```python
from build123d import *

# Parameters (mm, degrees)
F1_DEPTH = 12
F2_DEPTH = 8
F3_DEPTH = 5
F4_D     = 1.25


with BuildPart() as f1:
    # F0 (on Front) → F1 (new body)
    with BuildSketch(Plane.XZ):
        with BuildLine():
            Line((10.99224894, 5.3214330306), (12.920611769, 7.61956636))
            ThreePointArc((12.920611769, 7.61956636), (10.5696440554, 10.6434310512), (7.529497646, 12.9733058701))
            Line((7.529497646, 12.9733058701), (5.1924112184, 10.1880747237))
            Line((5.1924112184, 10.1880747237), (10.99224894, 5.3214330306))
        make_face()
        Polygon((3.2635182233, -3.8893095672), (10.99224894, 5.3214330306), (5.1924112184, 10.1880747237), (0, 4), (0, 0), align=None)
        Polygon((-3.939231012, -0.6945927107), (0, 0), (0, 4), align=None)
        Polygon((-3.3318045088, -11.7493091275), (3.2635182233, -3.8893095672), (0, 0), (-3.939231012, -0.6945927107), (-9.1316422304, -6.8826674344), align=None)
        with BuildLine():
            ThreePointArc((-11.4687286581, -9.6678985807), (-8.6463339891, -12.2572798185), (-5.2601673378, -14.0474424568))
            Line((-5.2601673378, -14.0474424568), (-3.3318045088, -11.7493091275))
            Line((-3.3318045088, -11.7493091275), (-9.1316422304, -6.8826674344))
            Line((-9.1316422304, -6.8826674344), (-11.4687286581, -9.6678985807))
        make_face()
    extrude(amount=F1_DEPTH)

    # F0 (on Front) → F2 (cut)
    with BuildSketch(Plane.XZ):
        Polygon((-3.939231012, -0.6945927107), (0, 0), (0, 4), align=None)
        Polygon((3.2635182233, -3.8893095672), (10.99224894, 5.3214330306), (5.1924112184, 10.1880747237), (0, 4), (0, 0), align=None)
        Polygon((-3.3318045088, -11.7493091275), (3.2635182233, -3.8893095672), (0, 0), (-3.939231012, -0.6945927107), (-9.1316422304, -6.8826674344), align=None)
    extrude(amount=F2_DEPTH, mode=Mode.SUBTRACT)

    # F0 (on Front) → F3 (join)
    with BuildSketch(Plane.XZ):
        with BuildLine():
            Line((5.1924112184, 10.1880747237), (7.529497646, 12.9733058701))
            ThreePointArc((7.529497646, 12.9733058701), (3.8987441535, 14.4844673366), (0, 15))
            Line((0, 15), (0, 4))
            Line((0, 4), (5.1924112184, 10.1880747237))
        make_face()
        Polygon((3.2635182233, -3.8893095672), (10.99224894, 5.3214330306), (5.1924112184, 10.1880747237), (0, 4), (0, 0), align=None)
        with BuildLine():
            Line((0, 4), (0, 15))
            ThreePointArc((0, 15), (-11.4906666468, 9.6418141453), (-14.7721162952, -2.604722665))
            Line((-14.7721162952, -2.604722665), (-3.939231012, -0.6945927107))
            Line((-3.939231012, -0.6945927107), (0, 4))
        make_face()
        with BuildLine():
            ThreePointArc((-14.7721162952, -2.604722665), (-13.5874059139, -6.3547148269), (-11.4687286581, -9.6678985807))
            Line((-11.4687286581, -9.6678985807), (-9.1316422304, -6.8826674344))
            Line((-9.1316422304, -6.8826674344), (-3.939231012, -0.6945927107))
            Line((-3.939231012, -0.6945927107), (-14.7721162952, -2.604722665))
        make_face()
        Polygon((-3.3318045088, -11.7493091275), (3.2635182233, -3.8893095672), (0, 0), (-3.939231012, -0.6945927107), (-9.1316422304, -6.8826674344), align=None)
        Polygon((-3.939231012, -0.6945927107), (0, 0), (0, 4), align=None)
        with BuildLine():
            ThreePointArc((9.6418141453, -11.4906666468), (13.5946168055, -6.3392739261), (15, 0))
            ThreePointArc((15, 0), (14.4708185072, 3.949102649), (12.920611769, 7.61956636))
            Line((12.920611769, 7.61956636), (10.99224894, 5.3214330306))
            Line((10.99224894, 5.3214330306), (3.2635182233, -3.8893095672))
            Line((3.2635182233, -3.8893095672), (9.6418141453, -11.4906666468))
        make_face()
        with BuildLine():
            ThreePointArc((-5.2601673378, -14.0474424568), (2.5365296809, -14.7839783948), (9.6418141453, -11.4906666468))
            Line((9.6418141453, -11.4906666468), (3.2635182233, -3.8893095672))
            Line((3.2635182233, -3.8893095672), (-3.3318045088, -11.7493091275))
            Line((-3.3318045088, -11.7493091275), (-5.2601673378, -14.0474424568))
        make_face()
    extrude(amount=F3_DEPTH)

    # F4 (through all)
    with Locations(Plane(origin=(0, 0, 0), x_dir=(1, 0, 0), z_dir=(0, 1, 0))):
        with Locations((7.3920575114, 8.8095110959), (-11.3252891596, 1.9969540432), (0, -11.5)):
            Hole(F4_D / 2)


solid = f1.part
```
The listing builds one solid part. Answer for the finished solid, in the listing's coordinates (mm). A direction names the side the tool comes from. Round coordinates to 2 decimals unless told otherwise and drop trailing zeros. Loops run counter-clockwise (first coordinate to the right, second up) from the corner with the lowest first, then second, coordinate; pieces in that order, holes last.
Q1. Which of the six approach directions +Z, -Z, +X, -X, +Y, -Y give full straight-line access (tool end or side, diameter ignored) to faces 5 (the face through (-6.272, -6.479, -9.282)), 6 (the face through (-10.7, -2.5, -2)), 7 (the face through (1, -8, -1))?
Q2. Section B-B, the plane y = -7.25 is taken. Determine the outline of the cut face in (x, z).
Q3. Given pin 1 Ø1.1 at (x, z) = (7.39, -8.81) entering from -Y; pin 2 Ø3 at (x, y) = (3, -2.5) entering from -Z; pin 3 Ø2 at (x, z) = (0, 11.5) entering from +Y; pin 4 Ø4 at (x, y) = (-9, -8) entering from -Z, each flat-ended and moving along its own axis, determine where each tip first touches the part or whether it passes through.
Q4. Find the intervals of material crossed by line 1 (Y direction, x = 2.5, z = 3.25); line 2 (Y direction, x = 10, z = 1.5); line 3 (X direction, y = -1.55, z = 11.5) (3 decimals), in increasing order.
Q5. For a pull along Y with two mould halves and no side action, classify faces 1 (the face through (8.133, -6.479, 7.721)), 2 (the face through (7.853, -2.535, -9.232)), 3 (the face through (0, -5, 0)), 4 (the face through (0, 0, 0)) as released by +Y, released by -Y, zero draft, split by the parting line, or undercut.
Q6. Section C-C, the plane x = -1 is taken. Determine the outline of the cut face in (y, z), then the cut area to 3 significant figures.
Q7. Section D-D, the plane y = -10.75 is taken. Determine the outline of the cut face in (x, z).
Q8. Section A-A, the plane z = 11.5 is taken. Determine the outline of the cut face in (x, y) (3 decimals).
Completed:
1. face 5: +Z, +X
1. face 6: +Y, -Y
1. face 7: none
2. outline: (-11.47, -9.67) arc R15 ccw to (-5.26, -14.05) - (-3.33, -11.75) - (-9.13, -6.88) - close; (5.19, 10.19) - (10.99, 5.32) - (12.92, 7.62) arc R15 ccw to (7.53, 12.97) - close
3. pin 1: passes through
3. pin 2: stops at z = -14.92
3. pin 3: stops at y = 0
3. pin 4: stops at z = -13.27
4. line 1: y = -12 to -8, -5 to 0
4. line 2: y = -5 to 0
4. line 3: x = -9.631 to -0.625, 0.625 to 9.631
5. face 1: undercut
5. face 2: zero draft
5. face 3: undercut
5. face 4: released by +Y
6. outline: (-12, -8.97) - (-8, -8.97) - (-8, 2.81) - (-12, 2.81) - close; (-5, -14.97) - (0, -14.97) - (0, 14.97) - (-5, 14.97) - close
6. area: 197 mm2
7. outline: (-11.47, -9.67) arc R15 ccw to (-5.26, -14.05) - (12.92, 7.62) arc R15 ccw to (7.53, 12.97) - close
8. outline: (-9.631, -5) - (-0.625, -5) - (-0.625, 0) - (-9.631, 0) - close; (0.625, -5) - (6.293, -5) - (6.293, -12) - (9.631, -12) - (9.631, 0) - (0.625, 0) - close
